Build history of the part. All positions in model axes, mm. A direction names the side the tool comes from. Give positions to 0.01 mm unless a question says otherwise; leave off trailing zeros. Loops run counter-clockwise (first coordinate to the right, second up) from the corner with the lowest first, then second, coordinate; pieces in that order, holes last.
1) Band-saw the part on B-B on y = -46.5. List the corners of the cut face in (x, z).
2) Band-saw the part on D-D on z = 21.5. List the corners of the cut face in (x, y), then the cut area to 3 significant figures.
3) Wall check: line 1 (Y direction, x = 40, z = 3.2); line 2 (Y direction, x = 4.4, z = 34.25); line 3 (Y direction, x = 76, z = 54.25). Give the ranges that are in metal, low to high.
4) Band-saw the part on C-C on x = 54.5. List the corners of the cut face in (y, z).
5) 3-axis set-ups, long thin cutter, end or side, ignore diameter. For faces 4 (the flat face through (73, -37, 57)), 5 (the cylindrical face through (61.423, -129.774, 8.697)), 6 (the flat face through (5, -51, 49)), 7 (the flat face through (23, -151, 16)): which of +Z, -Z, +X, -X, +Y, -Y reach the whole face in a straight line?
6) Band-saw the part on A-A on z = 43. State how many separate pieces and enclosed holes the cut face has, then the cut area to 3 significant figures.
7) Two-plate mould, pull along Y, no slides. Class faces 1 (the flat face through (16.5, -151, 22)), 2 (the flat face through (72, -77, 38)), 3 (the flat face through (4, -75, 60)): +Y half, -Y half, draft (parallel to the pull), parting line (faces both ways), or undercut.
8) Flat gauge pins, fed straight in: P1, Ø2, axis at x = 60.5, y = -128, coming from the +Z side; P2, Ø3.5, axis at x = 4, y = -79.5, coming from the +Z side; P3, Ø6.5, axis at x = 5.5, z = 60.5, coming from the -Y side. Where does each tip first touch, or does it go through?
Autodesk Inventor part; units mm, degrees
ref_plane "YZ Plane" through (0, 0, 0) normal (1, 0, 0) x (0, 1, 0)
ref_plane "XZ Plane" through (0, 0, 0) normal (0, 1, 0) x (-1, 0, 0)
ref_plane "XY Plane" through (0, 0, 0) normal (0, 0, 1) x (1, 0, 0)
sketch "Boceto1" plane through (0, 0, 0) normal (0, 0, 1) x (1, 0, 0)
  line L0 (0, 0) -> (80, 0)
  line L1 (80, 0) -> (80, -155)
  line L2 (80, -155) -> (0, -155)
  line L3 (0, -155) -> (0, 0)
  dimension "d0" = 155
  dimension "d1" = 80
extrude "Extrusión1" add sketch "Boceto1" along normal blind 82
sketch "Boceto2" plane through (0, 0, 82) normal (0, 0, 1) x (1, 0, 0)
  line L0 (8, -7.5) -> (72, -7.5)
  line L1 (72, -7.5) -> (72, -147.5)
  line L2 (72, -147.5) -> (8, -147.5)
  line L3 (8, -147.5) -> (8, -7.5)
  line L4 (80, -155) -> (80, 0)
  line L5 (0, 0) -> (0, -155)
  line L6 (80, 0) -> (0, 0)
  line L7 (0, -155) -> (80, -155)
  dimension "d4" = 8
  dimension "d5" = 8
  dimension "d6" = 7.5
  dimension "d7" = 7.5
  dimension "d8" = 64
  dimension "d9" = 140
extrude "Extrusión2" cut sketch "Boceto2" against normal blind 70 contours L0 L1 L2 L3
sketch "Boceto3" plane through (0, 0, 12) normal (0, 0, 1) x (1, 0, 0)
  line L0 (72, -147.5) -> (8, -147.5)
  line L1 (8, -147.5) -> (8, -7.5)
  line L2 (72, -7.5) -> (72, -147.5)
  line L3 (10, -142) -> (70, -142)
  circle A0 centre (12.5, -127) radius 2
  circle A1 centre (60.5, -128) radius 2
  circle A2 centre (60.5, -46.5) radius 2
  point P0 (0, 0)
  dimension "d20" = 60
  dimension "d21" = 2
  dimension "d22" = 2
  dimension "d23" = 5.5
  dimension "d24" = 15
  dimension "d25" = 14
  dimension "d26" = 4.5
  dimension "d27" = 11.5
  dimension "d28" = 95.5
  dimension "d29" = 11.5
  dimension "d30" = 4
extrude "Extrusión3" cut sketch "Boceto3" against normal blind 6.7
sketch "Boceto4" plane through (0, 0, 12) normal (0, 0, 1) x (1, 0, 0)
  line L0 (40, 12.201) -> (40, -183.6096)
  circle A0 centre (40, -57.5) radius 3
  circle A1 centre (40, -117.5) radius 3
  line L1 (72, -147.5) -> (8, -147.5)
  line L2 (0, -155) -> (80, -155)
  point P0 (0, 0)
  point P1 (40, -155)
  point P2 (40, -155)
  dimension "d33" = 60
  dimension "d34" = 6
  dimension "d35" = 30
  dimension "d103" = 0
extrude "Extrusión4" cut sketch "Boceto4" against normal through all
sketch "Boceto5" plane through (0, 0, 12) normal (0, 0, 1) x (1, 0, 0)
  circle A0 centre (40, -57.5) radius 3
  line L0 (45.9467, -57.5) -> (42.9734, -62.65)
  line L1 (42.9734, -62.65) -> (37.0266, -62.65)
  line L2 (37.0266, -62.65) -> (34.0533, -57.5)
  line L3 (34.0533, -57.5) -> (37.0266, -52.35)
  line L4 (37.0266, -52.35) -> (42.9734, -52.35)
  line L5 (42.9734, -52.35) -> (45.9467, -57.5)
  circle A1 centre (40, -117.5) radius 3
  line L6 (45.9467, -117.5) -> (42.9734, -122.65)
  line L7 (42.9734, -122.65) -> (37.0266, -122.65)
  line L8 (37.0266, -122.65) -> (34.0533, -117.5)
  line L9 (34.0533, -117.5) -> (37.0266, -112.35)
  line L10 (37.0266, -112.35) -> (42.9734, -112.35)
  line L11 (42.9734, -112.35) -> (45.9467, -117.5)
  point P0 (0, 0)
  dimension "d38" = 10.3
extrude "Extrusión5" cut sketch "Boceto5" against normal blind 6 contours A0 | L0 L1 L2 L3 L4 L5 | A1 | L6 L7 L8 L9 L10 L11
sketch "Boceto6" plane through (0, -155, 0) normal (0, -1, 0) x (1, 0, 0)
  line L0 (0, 0) -> (80, 0)
  line L1 (72, 12) -> (8, 12)
  line L2 (16.5, 16) -> (29.5, 16)
  line L3 (16.5, 28) -> (29.5, 28)
  line L4 (10, 12) -> (10, 44.9628)
  line L5 (70, 12) -> (70, 46.4487)
  line L6 (8, 82) -> (8, 12)
  line L7 (72, 82) -> (72, 12)
  line L8 (16.5, 28) -> (16.5, 16)
  line L9 (29.5, 28) -> (29.5, 16)
  line L10 (47, 45) -> (68.5, 45)
  line L11 (47, 28.5) -> (68.5, 28.5)
  line L12 (47, 28.5) -> (47, 45)
  line L13 (68.5, 28.5) -> (68.5, 45)
  point P0 (23, 16)
  dimension "d41" = 12
  dimension "d42" = 4
  dimension "d43" = 16
  dimension "d44" = 2
  dimension "d45" = 2
  dimension "d46" = 13
  dimension "d47" = 13
  dimension "d48" = 6.5
  dimension "d49" = 6.5
  dimension "d50" = 12
  dimension "d53" = 33
  dimension "d54" = 16.5
  dimension "d55" = 21.5
  dimension "d56" = 1.5
  dimension "d57" = 1.5
  dimension "d58" = 16.5
extrude "Extrusión6" cut sketch "Boceto6" against normal up to surface (7.5 mm away)
fillet "Empalme1" radius 4 4 edges at (47, -155, 36.75) (57.75, -155, 45) (68.5, -155, 36.75) (57.75, -155, 28.5)
sketch "Boceto8" plane through (72, -147.5, 82) normal (-1, 0, 0) x (0, 0, 1)
  line L0 (-50, 126.4237) -> (-50, 59.6822)
  line L1 (-70, 0) -> (-70, 140)
  circle A0 centre (-39, 136.5) radius 2
  circle A1 centre (-39, 110.5) radius 2
  line L2 (-54.9354, 5.5) -> (-15.6963, 5.5)
  line L3 (0, 0) -> (-70, 0)
  line L4 (-50, 108) -> (-15.6963, 108)
  line L5 (-50, 139) -> (-21.6523, 139)
  point P0 (-82, 147.5)
  dimension "d60" = 20
  dimension "d61" = 4
  dimension "d62" = 11
  dimension "d63" = 11
  dimension "d64" = 5.5
  dimension "d65" = 102.5
  dimension "d66" = 2.5
  dimension "d67" = 31
  dimension "d68" = 2.5
extrude "Extrusión7" cut sketch "Boceto8" against normal through all
sketch "Boceto9" plane through (8, -147.5, 82) normal (1, 0, 0) x (0, 0, -1)
  line L0 (50, 55) -> (50, 136)
  line L1 (70, 140) -> (70, 0)
  line L2 (29.5, 55) -> (29.5, 136)
  line L3 (50, 55) -> (29.5, 55)
  line L4 (29.5, 136) -> (50, 136)
  point P0 (82, 147.5)
  point P1 (0, 140)
  point P2 (39.75, 55)
  dimension "d71" = 20
  dimension "d72" = 20.5
  dimension "d73" = 81
  dimension "d75" = 4
  dimension "d101" = 30.25
extrude "Extrusión8" cut sketch "Boceto9" against normal blind 1.5
sketch "Boceto10" plane through (6.5, -147.5, 82) normal (1, 0, 0) x (0, 0, -1)
  line L0 (35, 59.5) -> (35, 131.5)
  line L1 (35, 131.5) -> (31, 131.5)
  line L2 (31, 131.5) -> (31, 59.5)
  line L3 (31, 59.5) -> (35, 59.5)
  line L4 (29.5, 55) -> (29.5, 136)
  line L5 (29.5, 136) -> (50, 136)
  point P0 (82, 147.5)
  point P1 (29.5, 95.5)
  dimension "d79" = 72
  dimension "d80" = 1.5
  dimension "d81" = 4
  dimension "d83" = 36
extrude "Extrusión9" cut sketch "Boceto10" against normal blind 1.5
sketch "Boceto11" plane through (6.5, -147.5, 82) normal (1, 0, 0) x (0, 0, -1)
  circle A0 centre (31.75, 57.5) radius 0.8
  circle A1 centre (47.75, 57.5) radius 0.8
  circle A2 centre (31.75, 133.5) radius 0.8
  circle A3 centre (47.75, 133.5) radius 0.8
  line L0 (50, 136) -> (50, 55)
  line L1 (50, 55) -> (29.5, 55)
  line L2 (29.5, 55) -> (29.5, 136)
  line L3 (29.5, 136) -> (50, 136)
  point P0 (82, 147.5)
  dimension "d86" = 1.6
  dimension "d88" = 2.25
  dimension "d89" = 2.25
  dimension "d91" = 2.5
  dimension "d92" = 2.25
  dimension "d93" = 2.5
  dimension "d94" = 2.5
  dimension "d95" = 2.5
  dimension "d96" = 2.25
extrude "Extrusión10" cut sketch "Boceto11" against normal blind 3.5 contours A0 | A1 | A2 | A3
sketch "Boceto12" plane through (0, 0, 82) normal (0, 0, 1) x (1, 0, 0)
  line L0 (0, -75) -> (80, -75)
  line L1 (0, -155) -> (80, -155)
  line L2 (0, -75) -> (0, -155)
  line L3 (0, -155) -> (80, -155)
  line L4 (80, -155) -> (80, -75)
  point P0 (0, 0)
  point P1 (40, -155)
  dimension "d99" = 80
  dimension "d100" = 40
  dimension "d104" = 80
  dimension "d105" = 80
extrude "Extrusión11" cut sketch "Boceto12" against normal blind 25
sketch "Boceto13" plane through (8, -7.5, 82) normal (0, -1, 0) x (1, 0, 0)
  line L0 (0, -70) -> (64, -70)
  circle A0 centre (32, -70) radius 17.5
  point P0 (-8, -82)
  point P1 (49.5, -70)
  point P2 (14.5, -70)
  dimension "d108" = 35
extrude "Extrusión12" cut sketch "Boceto13" against normal through all contours A0 L0 picked at (31.4056, -58.945)
sketch "Boceto14" plane through (0, 0, 57) normal (0, 0, 1) x (1, 0, 0)
  circle A0 centre (4, -150.5) radius 2
  circle A1 centre (4, -79.5) radius 2
  circle A2 centre (76, -79.5) radius 2
  circle A3 centre (76, -150.5) radius 2
  line L0 (80, -155) -> (0, -155)
  line L1 (0, -155) -> (0, -75)
  line L2 (0, -75) -> (8, -75)
  line L3 (80, -75) -> (80, -155)
  line L4 (72, -75) -> (80, -75)
  point P0 (0, 0)
  dimension "d111" = 4
  dimension "d112" = 4.5
  dimension "d113" = 4
  dimension "d114" = 4.5
  dimension "d115" = 4
  dimension "d116" = 4
  dimension "d117" = 4.5
  dimension "d118" = 4
  dimension "d119" = 4.5
extrude "Extrusión13" cut sketch "Boceto14" against normal blind 6.7
sketch "Boceto15" plane through (0, 0, 82) normal (0, 0, 1) x (1, 0, 0)
  line L0 (0, 0) -> (0, -75)
  line L1 (72, -75) -> (80, -75)
  line L2 (0, 0) -> (80, 0)
  line L3 (80, 0) -> (80, -75)
  line L4 (80, -75) -> (0, -75)
  line L5 (0, -75) -> (0, 0)
extrude "Extrusión14" cut sketch "Boceto15" against normal blind 19
fillet "Empalme2" radius 4 4 edges at (0, -155, 28.5) (80, -155, 28.5) (80, 0, 31.5) (0, 0, 31.5)
sketch "Boceto16" plane through (0, 0, 63) normal (0, 0, 1) x (1, 0, 0)
  line L0 (22.5, 0) -> (57.5, 0)
  line L1 (27.5, -7.5) -> (52.5, -7.5)
  line L2 (52.5, -7.5) -> (52.5, 0)
  line L3 (52.5, 0) -> (27.5, 0)
  line L4 (27.5, 0) -> (27.5, -7.5)
  line L5 (8, -147.5) -> (8, -7.5)
  line L6 (0, -25) -> (8, -25)
  line L7 (8, -25) -> (8, -50)
  line L8 (8, -50) -> (0, -50)
  line L9 (0, -50) -> (0, -25)
  line L10 (8, -75) -> (0, -75)
  line L11 (40, 16.6758) -> (40, -44.6226)
  line L12 (80, -25) -> (72, -25)
  line L13 (72, -25) -> (72, -50)
  line L14 (72, -50) -> (80, -50)
  line L15 (80, -50) -> (80, -25)
  point P0 (40, 0)
  dimension "d129" = 25
  dimension "d130" = 7.5
  dimension "d131" = 12.5
  dimension "d132" = 8
  dimension "d133" = 25
  dimension "d134" = 25
extrude "Extrusión15" cut sketch "Boceto16" against normal blind 6
sketch "Boceto17" plane through (0, 0, 57) normal (0, 0, 1) x (1, 0, 0)
  circle A0 centre (40, -3.75) radius 2
  circle A1 centre (4, -37.5) radius 2
  line L0 (5, -77.7679) -> (5, -16)
  circle A2 centre (76, -37.5) radius 2
  line L1 (0, -50) -> (0, -25)
  line L2 (0, -25) -> (8, -25)
  line L3 (80, -50) -> (72, -50)
  line L4 (80, -25) -> (80, -50)
  line L5 (52.5, -7.5) -> (27.5, -7.5)
  line L6 (27.5, -7.5) -> (27.5, 0)
  point P0 (0, 0)
  dimension "d137" = 4
  dimension "d138" = 4
  dimension "d139" = 12.5
  dimension "d140" = 12.5
  dimension "d141" = 4
  dimension "d142" = 3.75
  dimension "d143" = 12.5
extrude "Extrusión16" cut sketch "Boceto17" against normal blind 6.7
properties part number "Caja para Electrónica"
Findings below:
1. outline: (0, 0) - (80, 0) - (80, 57) - (72, 57) - (72, 12) - (62.5, 12) - (62.5, 5.3) - (58.5, 5.3) - (58.5, 12) - (8, 12) - (8, 32) - (6.5, 32) - (6.5, 47) - (5, 47) - (5, 51) - (6.5, 51) - (6.5, 52.5) - (8, 52.5) - (8, 57) - (0, 57) - close
2. outline: (0, -151) arc R4 ccw to (4, -155) - (16.5, -155) - (16.5, -147.5) - (8, -147.5) - (8, -7.5) - (25.3, -7.5) - (25.3, 0) - (4, 0) arc R4 ccw to (0, -4) - close; (29.5, -155) - (76, -155) arc R4 ccw to (80, -151) - (80, -4) arc R4 ccw to (76, 0) - (54.7, 0) - (54.7, -7.5) - (72, -7.5) - (72, -147.5) - (29.5, -147.5) - close
2. area: 3,110 mm2
3. line 1: y = -155 to -120.5, -114.5 to -60.5, -54.5 to 0
3. line 2: y = -155 to -90.8, -89.2 to -14.8, -13.2 to 0
3. line 3: y = -155 to -152.5, -148.5 to -81.5, -77.5 to -39.5, -35.5 to 0
4. outline: (-155, 0) - (0, 0) - (0, 12) - (-147.5, 12) - (-147.5, 28.5) - (-151, 28.5) arc R4 ccw to (-155, 24.5) - close; (-155, 49) arc R4 ccw to (-151, 45) - (-147.5, 45) - (-147.5, 57) - (-155, 57) - close; (-7.5, 21.8) - (0, 21.8) - (0, 63) - (-7.5, 63) - close
5. face 4: +Z, +X, -X
5. face 5: +Z
5. face 6: none
5. face 7: -Y
6. separate pieces: 3
6. enclosed holes: 0
6. area: 3,070 mm2
7. face 1: draft
7. face 2: undercut
7. face 3: -Y half
8. P1: stops at z = 5.3
8. P2: stops at z = 50.3
8. P3: stops at y = -75
